Autodesk Inventor part; units mm, degrees
ref_plane "YZ Plane" through (0, 0, 0) normal (1, 0, 0) x (0, 1, 0)
ref_plane "XZ Plane" through (0, 0, 0) normal (0, 1, 0) x (-1, 0, 0)
ref_plane "XY Plane" through (0, 0, 0) normal (0, 0, 1) x (1, 0, 0)
sketch "Sketch1" plane through (0, 0, 0) normal (0, 0, 1) x (1, 0, 0)
  line L0 (-15.561, 10.0244) -> (24.939, 10.0244)
  line L1 (24.939, 10.0244) -> (24.939, -9.9756)
  line L2 (24.939, -9.9756) -> (-15.561, -9.9756)
  line L3 (-15.561, -9.9756) -> (-15.561, 10.0244)
  point P0 (0, 0)
  dimension "d0" = 20
  dimension "d1" = 40.5
extrude "Extrusion1" add sketch "Sketch1" along normal blind 36.1
sketch "Sketch2" plane through (24.939, -9.9756, 0) normal (1, 0, 0) x (0, 0, -1)
  line L0 (-36.1, 20) -> (-36.1, 0)
  line L1 (-36.1, 13.8904) -> (-32.1201, 13.8904)
  line L2 (-32.1201, 13.8904) -> (-32.1201, 5.486)
  line L3 (-32.1201, 5.486) -> (-36.1, 5.486)
  line L4 (-36.1, 5.486) -> (-36.1, 13.8904)
  point P0 (0, 9.9756)
extrude "Extrusion2" add sketch "Sketch2" along normal blind 5.08
sketch "Sketch3" plane through (24.939, -9.9756, 0) normal (1, 0, 0) x (0, 0, -1)
  line L0 (-36.1, 13.8904) -> (-36.1, 20)
  line L1 (-7.2964, 16.9452) -> (-7.2964, 3.5991)
  line L2 (-9.7348, 3.5991) -> (-9.7348, 16.9452)
  line L3 (-9.7348, 16.9452) -> (-9.7348, 20)
  line L4 (0, 20) -> (-36.1, 20)
  line L5 (-7.2964, 16.9452) -> (-7.2964, 20)
  line L6 (-7.2964, 3.5991) -> (-7.2964, 0)
  line L7 (0, 0) -> (-36.1, 0)
  line L8 (-9.7348, 3.5991) -> (-9.7348, 0)
  point P0 (0, 9.9756)
extrude "Extrusion3" add sketch "Sketch3" along normal blind 8.0264
sketch "Sketch4" plane through (-15.561, -9.9756, 0) normal (-1, 0, 0) x (0, 0, 1)
  line L0 (0, 0) -> (7.2964, 0)
  line L1 (9.7348, 20) -> (36.1, 20)
  line L2 (7.2964, 0) -> (9.7348, 0)
  line L3 (9.7348, 0) -> (9.7348, 20)
  line L4 (9.7348, 20) -> (7.2964, 20)
  line L5 (7.2964, 20) -> (7.2964, 0)
  point P0 (0, 9.9756)
extrude "Extrusion4" add sketch "Sketch4" along normal blind 8.0264
sketch "Sketch5" plane through (24.939, -9.9756, 7.2964) normal (0, 0, -1) x (-1, 0, 0)
  line L0 (0, 20) -> (-8.0264, 20)
  circle A0 centre (-5.1734, 4.773) radius 2.3347
  line L1 (40.5, 0) -> (48.5264, 0)
  line L2 (40.5, 20) -> (48.5264, 20)
  circle A1 centre (45.3266, 4.773) radius 2.3347
  circle A2 centre (45.3266, 15.1496) radius 2.3347
  circle A3 centre (-5.1734, 15.1496) radius 2.3347
  point P0 (24.939, 9.9756)
  dimension "d18" = 50.5
hole "Hole1" at (30.1124, -5.2026, 7.2964) at (30.1124, 5.174, 7.2964) at (-20.3876, -5.2026, 7.2964) at (-20.3876, 5.174, 7.2964) direction (0, 0, 1) diameter 4.7625 end through all
sketch "Sketch6" plane through (0, 0, 0) normal (0, 0, -1) x (-1, 0, 0)
  line L0 (15.561, -9.9756) -> (15.561, 10.0244)
  line L1 (15.561, 0.0244) -> (-14.839, 0.0244)
  circle A0 centre (-14.839, 0.0244) radius 2.9972
  point P0 (0, 0)
  dimension "d26" = 30.4
  dimension "d27" = 5.9944
extrude "Extrusion5" add sketch "Sketch6" along normal blind 5.9944
sketch "Sketch7" plane through (0, 0, 36.1) normal (0, 0, 1) x (1, 0, 0)
  point P0 (0, 0)
sketch "Sketch8" plane through (0, 0, 0) normal (0, 0, -1) x (-1, 0, 0)
  line L0 (15.561, -9.9756) -> (15.561, 10.0244)
  circle A0 centre (20.3876, -5.2026) radius 2.3813
  line L1 (15.561, -9.9756) -> (23.5874, -9.9756)
  point P0 (0, 0)
  dimension "d30" = 4.8266
  dimension "d31" = 4.7625
  dimension "d33" = 4.773
properties part number "Aidan Sherry Servo motor"
Work out the finished part from the listing and answer in its coordinate system (mm). A direction names the side the tool comes from. Give positions to 0.01 mm unless a question says otherwise; leave off trailing zeros. Loops run counter-clockwise (first coordinate to the right, second up) from the corner with the lowest first, then second, coordinate; pieces in that order, holes last. Notation, with made-up numbers: (-6, -26) -> (31, -26) arc R34 ccw to (31, 13) -> close; hole circle Ø7 at (36, 7.25). An arc over 180 degrees is marked (long way). Put each result on its own line as item: value. Start each with the question number.
Item 1: The part is cut by section C-C (z = 9). Give the vertices of the cut face in (x, y).
Item 2: Which of the six approach directions +Z, -Z, +X, -X, +Y, -Y give full straight-line access (tool end or side, diameter ignored) to faces 5 (the face through (-20, 0, 7.296)), 6 (the face through (26, 3.915, 34)), 7 (the face through (29, 0, 9.735)), 8 (the face through (-15.561, 0, 23))?
Item 3: Find the intervals of material crossed by L1, parallel to Y at x = -19.5, z = 7.5; L2, parallel to X at y = -6.5, z = 3.5; L3, parallel to X at y = 1.5, z = 33.5, in increasing order. Write a range as [from, to].
Item 4: The part is cut by section D-D (y = -3.75). Give the vertices of the cut face in (x, z), then the cut area to 3 significant figures.
Item 5: The part is cut by section B-B (y = -8.25). Give the vertices of the cut face in (x, z), then the cut area to 3 significant figures.
Item 6: The mould has two halves that part along X. Classify faces 1 (the face through (32.437, -5.719, 8.533)), 2 (the face through (32.437, 4.658, 8.533)), 3 (the face through (5, -9.976, 18)), 4 (the face through (24.939, 0, 4)): released by +X, released by -X, zero draft, split by the parting line, or undercut.
Item 7: The part is cut by section A-A (x = 27). Give the vertices of the cut face in (y, z), then the cut area to 3 significant figures.
Item 8: Each of these flat-tipped pins is pushed along its axis until it touches: P1, Ø6, axis at y = -4, z = 2, coming from the +X side; P2, Ø8, axis at y = 4.5, z = 2.5, coming from the -X side; P3, Ø6, axis at x = -4, y = 4.5, coming from the -Z side. Where does it stop, or does it pass through?
Answers below:
1. outline: (-23.59, -9.98) -> (32.97, -9.98) -> (32.97, 10.02) -> (-23.59, 10.02) -> close; hole circle Ø4.76 at (-20.39, -5.2); hole circle Ø4.76 at (-20.39, 5.17); hole circle Ø4.76 at (30.11, -5.2); hole circle Ø4.76 at (30.11, 5.17)
2. face 5: -Z, -X, +Y, -Y
2. face 6: +Z, +X, +Y
2. face 7: +X, +Y, -Y
2. face 8: +Z, -X, +Y, -Y
3. L1: [-9.98, -7.41], [-2.99, 2.96], [7.38, 10.02]
3. L2: [-15.56, 24.94]
3. L3: [-15.56, 30.02]
4. outline: (-23.59, 7.3) -> (-22.27, 7.3) -> (-22.27, 9.73) -> (-23.59, 9.73) -> close; (-18.5, 7.3) -> (-15.56, 7.3) -> (-15.56, 0) -> (24.94, 0) -> (24.94, 7.3) -> (28.23, 7.3) -> (28.23, 9.73) -> (24.94, 9.73) -> (24.94, 32.12) -> (28.23, 32.12) -> (28.23, 36.1) -> (-15.56, 36.1) -> (-15.56, 9.73) -> (-18.5, 9.73) -> close; (32, 7.3) -> (32.97, 7.3) -> (32.97, 9.73) -> (32, 9.73) -> close
4. area: 1,500 mm2
5. outline: (-23.59, 7.3) -> (-15.56, 7.3) -> (-15.56, 0) -> (24.94, 0) -> (24.94, 7.3) -> (32.97, 7.3) -> (32.97, 9.73) -> (24.94, 9.73) -> (24.94, 36.1) -> (-15.56, 36.1) -> (-15.56, 9.73) -> (-23.59, 9.73) -> close
5. area: 1,500 mm2
6. face 1: undercut
6. face 2: undercut
6. face 3: zero draft
6. face 4: released by +X
7. outline: (-9.98, 7.3) -> (10.02, 7.3) -> (10.02, 9.73) -> (-9.98, 9.73) -> close; (-4.49, 32.12) -> (3.91, 32.12) -> (3.91, 36.1) -> (-4.49, 36.1) -> close
7. area: 82.2 mm2
8. P1: x = 24.94
8. P2: x = -15.56
8. P3: z = 0
